Read the model definition and answer for the solid it produces. Units are mm, in the model's axes. Face numbers are marked on the shaded views. A direction names the side the tool comes from. Give positions to 0.01 mm unless a question says otherwise; leave off trailing zeros. Write each loop counter-clockwise with the first axis right and the second up, starting at its lowest first coordinate (ties: lowest second). Pieces come first, ordered by that corner, then holes. Notation, with made-up numbers: (-37, 38) - (19, 38) arc R35 cw to (19, 72) - close; hole circle Ø3 at (19, -26). An arc over 180 degrees is marked (long way). Use CSV: the item, a comma, the result in double quotes. Start each with the question number.
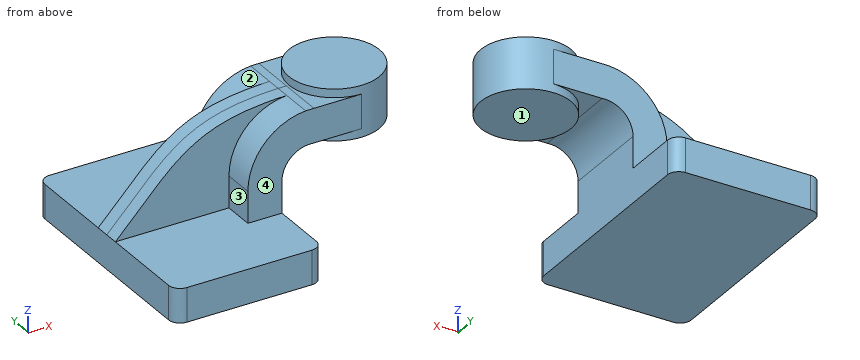
from build123d import *

# Parameters (mm, degrees)
F1_DEPTH = 63.5
F2_DEPTH = 25.4
F3_DEPTH = 7.9375
F0_W     = 25.4945200562
F0_H     = 19.05
F4_DEPTH = 25.4
F6_R     = 6.35


with BuildPart() as f1:
    # F0 (on Front) → F1 (new body, symmetric)
    with BuildSketch(Plane.XZ):
        Polygon((41.275, -9.525), (41.275, 9.525), (22.225, 9.525), (-41.275, 9.525), (-41.275, -9.525), align=None)
    extrude(amount=F1_DEPTH, both=True)

    # F0 (on Front) → F2 (join, symmetric)
    with BuildSketch(Plane.XZ):
        with BuildLine():
            Line((22.225, 9.525), (41.275, 9.525))
            Line((41.275, 9.525), (41.275, 27.0584095458))
            ThreePointArc((41.275, 27.0584095458), (46.4156191601, 38.7540793849), (58.5082211633, 42.8752))
            Line((58.5082211633, 42.8752), (60.325, 42.8752))
            Line((60.325, 42.8752), (60.325, 61.9252))
            Line((60.325, 61.9252), (59.1655764496, 61.9252))
            add(Edge.make_bspline(
                [(54.5329264401, 61.8852174814), (56.041241649, 61.9118488453), (57.5849624427, 61.9252), (59.1655764496, 61.9252)],
                knots=[110.2611541265, 110.2611541265, 110.2611541265, 110.2611541265, 113.2876443288, 113.2876443288, 113.2876443288, 113.2876443288], degree=3))
            ThreePointArc((54.5329264401, 61.8852174814), (31.5457335676, 50.8108234328), (22.225, 27.0584095458))
            Line((22.225, 27.0584095458), (22.225, 9.525))
        make_face()
    extrude(amount=F2_DEPTH, both=True)

    # F0 (on Front) → F3 (join, symmetric)
    with BuildSketch(Plane.XZ):
        with BuildLine():
            Line((-41.275, 9.525), (22.225, 9.525))
            Line((22.225, 9.525), (22.225, 27.0584095458))
            ThreePointArc((22.225, 27.0584095458), (31.5457335676, 50.8108234328), (54.5329264401, 61.8852174814))
            add(Edge.make_bspline(
                [(-41.275, 9.525), (-8.3754615169, 42.3180313799), (-0.4180446882, 60.9149830772), (54.5329264401, 61.8852174814)],
                knots=[0, 0, 0, 0, 110.2611541265, 110.2611541265, 110.2611541265, 110.2611541265], degree=3))
        make_face()
    extrude(amount=F3_DEPTH, both=True)

    # F0 (on Front) → F4 (join, symmetric)
    with BuildSketch(Plane.XZ):
        with Locations((73.0722600281, 52.4002)):
            Rectangle(F0_W, F0_H)
    extrude(amount=F4_DEPTH, both=True)

    # F0 (on Front) → F5 (revolve)
    with BuildSketch(Plane.XZ):
        Polygon((85.8195200562, 61.9252), (85.8195200562, 42.8752), (85.8195200562, 38.1), (111.125, 38.1), (111.125, 66.675), (85.8195200562, 66.675), align=None)
    revolve(axis=Axis((85.8195200562, 0, 52.3875), (0, 0, 1)))

    # F6
    f6_edges = [f1.edges().sort_by_distance(p)[0] for p in [
        (41.275, -63.5, 0),
        (-41.275, -63.5, 0),
        (41.275, 63.5, 0),
        (-41.275, 63.5, 0),
    ]]
    fillet(f6_edges, radius=F6_R)


solid = f1.part
(1) The part is cut by section A-A on x = 62.5. Write down the section's boundary in (y, z) (3 decimals), plus the area to 3 significant figures.
(2) Consider probe 1 along Z at (x, y) = (90, -20.5) (3 decimals); probe 2 along Z at (x, y) = (22, -39.5) (3 decimals); probe 3 along X at (y, z) = (-6.5, 2) (3 decimals). Determine where each line is inside the solid, lowest interval first.
(3) Which of the six approach directions +Z, -Z, +X, -X, +Y, -Y give full straight-line access (tool end or side, diameter ignored) to the marked faces 1, 2, 3 and 4?
(4) Given P1, Ø10, axis at x = 0.5, z = 57.5, coming from the -Y side; P2, Ø6, axis at x = 48.5, y = 25.5, coming from the +Z side; P3, Ø2, axis at y = 11.5, z = 45, coming from the -X side; P4, Ø1.5, axis at y = -26, z = 55, coming from the -X side, each flat-ended and moving along its own axis, determine where each tip first touches the part or whether it passes through.
Reported:
1,outline,"(-25.4, 42.875) - (-9.827, 42.875) - (-9.827, 38.1) - (9.827, 38.1) - (9.827, 42.875) - (25.4, 42.875) - (25.4, 61.925) - (9.827, 61.925) - (9.827, 66.675) - (-9.827, 66.675) - (-9.827, 61.925) - (-25.4, 61.925) - close"
1,area,"1,150 mm²"
2,probe 1,"38.1 to 66.675"
2,probe 2,"-9.525 to 9.525"
2,probe 3,"-41.275 to 41.275"
3,face 1,"-Z, +X, +Y, -Y"
3,face 2,"+Z, -X, +Y"
3,face 3,"+Z, -X, -Y"
3,face 4,"+Z, +X, -X, -Y"
4,P1,"through"
4,P2,"z = 61.52"
4,P3,"x = 26.61"
4,P4,"x = 35.61"
